Read the model definition and answer for the solid it produces. Units are mm, in the model's axes. Face numbers are marked on the shaded views. Give positions to 0.01 mm unless a question says otherwise; leave off trailing zeros. Write each loop counter-clockwise with the first axis right and the second up, starting at its lowest first coordinate (ties: lowest second). Pieces come first, ordered by that corner, then holes. Notation, with made-up numbers: M 38,46.25 L 42,46.25 A19 ccw 42,65.25 Z; hole C 35.25,68.25 d4. An arc over 180 degrees is marked long. Use a Markdown table: item, result. Add a question column.
Item 1: A cutting plane is placed at C-C on x = 3.25. Determine the outline of the cut face in (y, z).
Item 2: The mould has two halves that part along Z. Classify the marked faces 1, 2 and 3: pulls with the +Z half, pulls with the -Z half, needs draft (parallel to the pull), parting line crosses it, or undercut.
Item 3: A cutting plane is placed at A-A on z = 0. Determine the outline of the cut face in (x, y).
Item 4: A cutting plane is placed at D-D on z = 8. Determine the outline of the cut face in (x, y), then the cut area to 3 significant figures.
Item 5: Given P1, Ø6, axis at x = 3.5, z = -16, coming from the +Y side; P2, Ø1, axis at x = 5.5, z = 14.5, coming from the +Y side; P3, Ø9.5, axis at y = 8, z = 8, coming from the +X side; P4, Ø5, axis at x = 6.5, y = -4, coming from the -Z side, each flat-ended and moving along its own axis, determine where each tip first touches the part or whether it passes through.
Item 6: Consider probe 1 along Y at (x, z) = (4.5, -8); probe 2 along X at (y, z) = (-10, -10). Determine where each line is inside the solid, lowest interval first. Write a range as [from, to].
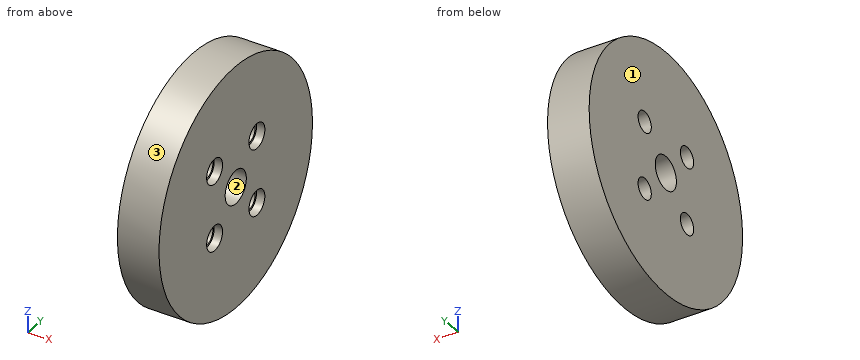
Autodesk Inventor part; units mm, degrees
ref_plane "YZ Plane" through (0, 0, 0) normal (1, 0, 0) x (0, 1, 0)
ref_plane "XZ Plane" through (0, 0, 0) normal (0, 1, 0) x (-1, 0, 0)
ref_plane "XY Plane" through (0, 0, 0) normal (0, 0, 1) x (1, 0, 0)
sketch "Sketch1" plane through (0, 0, 0) normal (1, 0, 0) x (0, 1, 0)
  circle A0 centre (0, 0) radius 29
  circle A1 centre (0, 0) radius 29
  dimension "d0" = 58
  dimension "d22" = 58
extrude "Extrusion1" add sketch "Sketch1" along normal blind 10
sketch "Sketch2" plane through (10, 0, 0) normal (1, 0, 0) x (0, 0, -1)
  point P0 (0, 0)
  point P1 (-8, 8)
  point P2 (8, 8)
  point P3 (8, -8)
  point P4 (-8, -8)
  dimension "d3" = 8
  dimension "d4" = 8
  dimension "d5" = 16
  dimension "d6" = 16
hole "Hole1" at (10, 8, 8) at (10, 8, -8) at (10, -8, -8) at (10, -8, 8) direction (-1, 0, 0) diameter 5 end through all counterbore diameter 6 counterbore depth 2
sketch "Sketch3" plane through (10, 0, 0) normal (1, 0, 0) x (0, 0, -1)
  point P0 (0, 0)
  point P1 (0, 0)
hole "Hole2" at (10, 0, 0) direction (-1, 0, 0) diameter 8 end through all
equation "\"d0\" = d22"
properties part number "Tapon 1_Cabeza"
Filled in:
| question | item | result |
|---|---|---|
| 1 | outline | C 0,0 d58; hole C -8,-8 d5; hole C -8,8 d5; hole C 0,0 d8; hole C 8,-8 d5; hole C 8,8 d5 |
| 2 | face 1 | needs draft |
| 2 | face 2 | undercut |
| 2 | face 3 | parting line crosses it |
| 3 | outline | M 0,-29 L 10,-29 L 10,-4 L 0,-4 Z; M 0,4 L 10,4 L 10,29 L 0,29 Z |
| 4 | outline | M 0,-27.87 L 10,-27.87 L 10,-11 L 8,-11 L 8,-10.5 L 0,-10.5 Z; M 0,-5.5 L 8,-5.5 L 8,-5 L 10,-5 L 10,5 L 8,5 L 8,5.5 L 0,5.5 Z; M 0,10.5 L 8,10.5 L 8,11 L 10,11 L 10,27.87 L 0,27.87 Z |
| 4 | area | 453 mm² |
| 5 | P1 | y = 25.92 |
| 5 | P2 | y = 25.4 |
| 5 | P3 | x = 10 |
| 5 | P4 | z = -28.96 |
| 6 | probe 1 | [-27.87, -10.5], [-5.5, 5.5], [10.5, 27.87] |
| 6 | probe 2 | [0, 8] |
